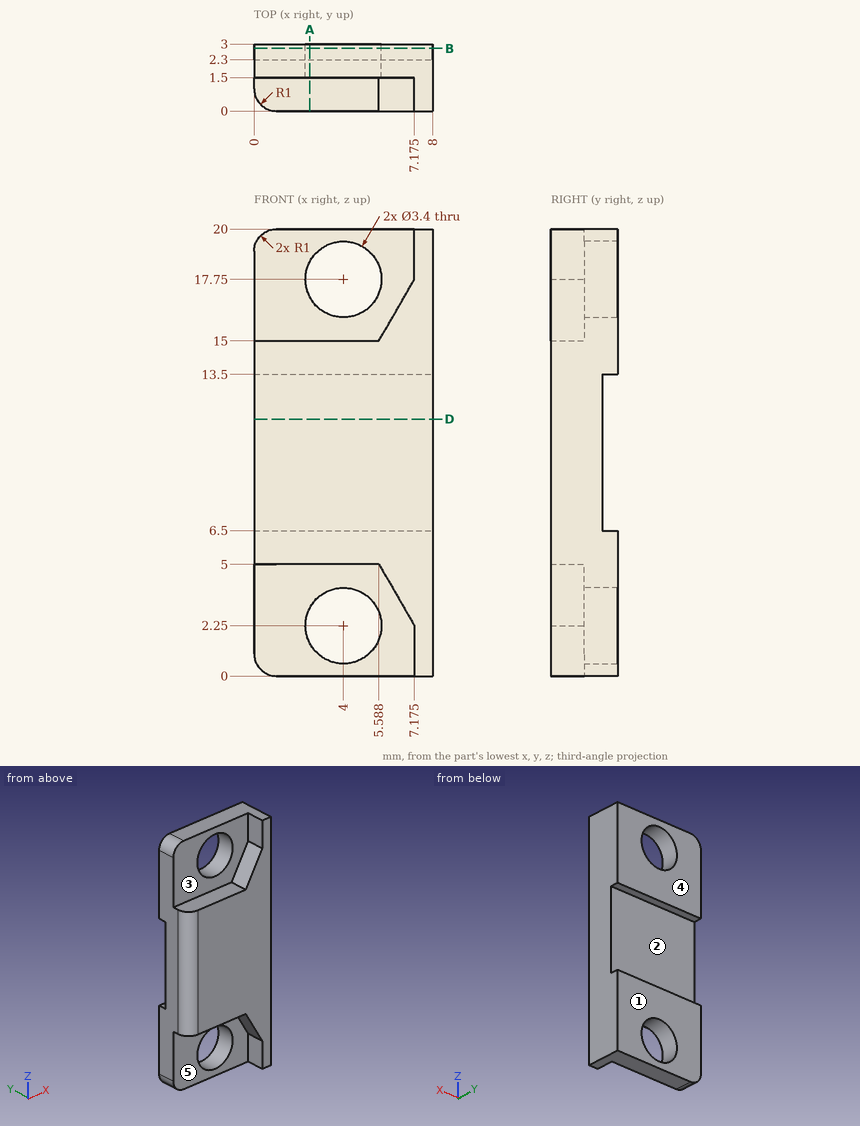
Print and shaded views of the part. All mm, measured from the part's lowest x, y and z. A direction names the side the tool comes from. Give positions to 0.01 mm unless a question says otherwise; leave off trailing zeros. Loops run counter-clockwise (first coordinate to the right, second up) from the corner with the lowest first, then second, coordinate; pieces in that order, holes last. Notation, with made-up numbers: (-5, 54) -> (49, 54) arc R23 cw to (49, 84) -> close; hole circle Ø6 at (-37.5, -7.5). An arc over 180 degrees is marked (long way). Use CSV: the item, a comma, the result in double quotes. Start each with the question number.
1) Mould opens along Z. For the marked faces 1 and 2 say: released by +Z, released by -Z, zero draft, split by the parting line, or undercut.
2) Wall check: line 1 (Z direction, x = 4, y = 2.1); line 2 (Z direction, x = 4, y = 2.45); line 3 (Y direction, x = 2, z = 11). Give the ranges that are in metal, low to high.
3) Slice it at D-D on z = 11.5. Give the cut face in (x, y), plus the area to 3 significant figures.
4) Slice it at B-B on y = 2.8. Give the cut face in (x, z).
5) Tool access for the marked faces 3, 4 and 5: list every direction of +Z, -Z, +X, -X, +Y, -Y with a clear straight run to the whole face (end or side of a thin tool).
6) Flat gauge pins, fed straight in: pin 1 Ø4 at (x, z) = (3.5, 18) entering from -Y; pin 2 Ø2 at (x, z) = (3, 11) entering from +Y; pin 3 Ø1.6 at (y, z) = (0.5, 1) entering from -X (1 decimal). Where does each tip first touch, or does it go through?
7) Slice it at A-A on x = 2.5. Give the cut face in (y, z).
Computed values:
1,face 1,"zero draft"
1,face 2,"undercut"
2,line 1,"z = 0 to 0.55, 3.95 to 16.05, 19.45 to 20"
2,line 2,"z = 0 to 0.55, 3.95 to 6.5, 13.5 to 16.05, 19.45 to 20"
2,line 3,"y = 0 to 2.3"
3,outline,"(0, 1) arc R1 ccw to (1, 0) -> (8, 0) -> (8, 2.3) -> (0, 2.3) -> close"
3,area,"18.2 mm^2"
4,outline,"(0, 1) arc R1 ccw to (1, 0) -> (8, 0) -> (8, 6.5) -> (0, 6.5) -> close; (0, 13.5) -> (8, 13.5) -> (8, 20) -> (1, 20) arc R1 ccw to (0, 19) -> close; hole circle Ø3.4 at (4, 2.25); hole circle Ø3.4 at (4, 17.75)"
5,face 3,"+Z, -X, -Y"
5,face 4,"+Z, -Z, +X, -X, +Y"
5,face 5,"-Z, -X, -Y"
6,pin 1,"stops at y = 1.5"
6,pin 2,"stops at y = 2.3"
6,pin 3,"stops at x = 7.2"
7,outline,"(0, 5) -> (1.5, 5) -> (1.5, 3.05) -> (3, 3.05) -> (3, 6.5) -> (2.3, 6.5) -> (2.3, 13.5) -> (3, 13.5) -> (3, 16.95) -> (1.5, 16.95) -> (1.5, 15) -> (0, 15) -> close; (1.5, 0) -> (3, 0) -> (3, 1.45) -> (1.5, 1.45) -> close; (1.5, 18.55) -> (3, 18.55) -> (3, 20) -> (1.5, 20) -> close"
